from build123d import *

# Parameters (mm, degrees)
SKETCH_R  = 1.75
PAD_DEPTH = 9
FILLET_R  = 2


with BuildPart() as part:
    # Sketch → Pad (new body)
    with BuildSketch(Plane.XY):
        with BuildLine():
            Line((-15, 16), (15, 16))
            ThreePointArc((19, 12), (17.828427, 14.828427), (15, 16))
            Line((19, 12), (19, -12))
            ThreePointArc((15, -16), (17.828427, -14.828427), (19, -12))
            Line((15, -16), (-15, -16))
            ThreePointArc((-19, -12), (-17.828427, -14.828427), (-15, -16))
            Line((-19, -12), (-19, 12))
            ThreePointArc((-15, 16), (-17.828427, 14.828427), (-19, 12))
        make_face()
        with Locations((-15, 12)):
            Circle(SKETCH_R, mode=Mode.SUBTRACT)
        with Locations((15, 12)):
            Circle(SKETCH_R, mode=Mode.SUBTRACT)
        with Locations((15, -12)):
            Circle(SKETCH_R, mode=Mode.SUBTRACT)
        with Locations((-15, -12)):
            Circle(SKETCH_R, mode=Mode.SUBTRACT)
        with BuildLine():
            Line((-16.75, 8), (-15, 8))
            ThreePointArc((-15, 8), (-12.171573, 9.171573), (-11, 12))
            Line((-11, 12), (-11, 13.75))
            Line((-11, 13.75), (11, 13.75))
            Line((11, 13.75), (11, 12))
            ThreePointArc((11, 12), (12.171573, 9.171573), (15, 8))
            Line((15, 8), (16.75, 8))
            Line((16.75, 8), (16.75, -8))
            Line((15, -8), (16.75, -8))
            ThreePointArc((15, -8), (12.171573, -9.171573), (11, -12))
            Line((11, -13.75), (11, -12))
            Line((11, -13.75), (-11, -13.75))
            Line((-11, -12), (-11, -13.75))
            ThreePointArc((-11, -12), (-12.171573, -9.171573), (-15, -8))
            Line((-16.75, -8), (-15, -8))
            Line((-16.75, -8), (-16.75, 8))
        make_face(mode=Mode.SUBTRACT)
    extrude(amount=PAD_DEPTH)

    # Fillet
    fillet_edges = [part.edges().sort_by_distance(p)[0] for p in [
        (-11, 13.75, 4.5),
        (-16.75, 8, 4.5),
        (11, 13.75, 4.5),
        (16.75, 8, 4.5),
        (16.75, -8, 4.5),
        (11, -13.75, 4.5),
        (-11, -13.75, 4.5),
        (-16.75, -8, 4.5),
    ]]
    fillet(fillet_edges, radius=FILLET_R)


solid = part.part
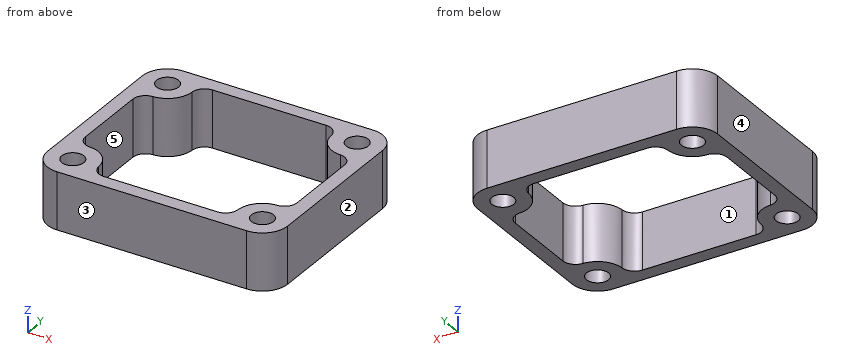
Work out the finished part from the listing and answer in its coordinate system (mm). Face numbers are marked on the shaded views. A direction names the side the tool comes from. Round coordinates to 2 decimals unless told otherwise and drop trailing zeros. Write each loop counter-clockwise with the first axis right and the second up, starting at its lowest first coordinate (ties: lowest second). Pieces come first, ordered by that corner, then holes. Notation, with made-up numbers: M -40,60.5 L -15,60.5 A34 cw -15,91.5 Z; hole C 88,15 d8. An arc over 180 degrees is marked long. Use a Markdown table: item, result.
1) Which of the six approach directions +Z, -Z, +X, -X, +Y, -Y give full straight-line access (tool end or side, diameter ignored) to the marked faces 1 and 2?
Taken from the geometry:
| item | result |
|---|---|
| face 1 | +Z, -Z |
| face 2 | +Z, -Z, +X, +Y, -Y |
2) The part is cut by section A-A on x = 7. Give the vertices of the cut face in (y, z), plus the area to 3 significant figures.
Taken from the geometry:
| item | result |
|---|---|
| outline | M -16,0 L -13.75,0 L -13.75,9 L -16,9 Z; M 13.75,0 L 16,0 L 16,9 L 13.75,9 Z |
| area | 40.5 mm2 |
3) The part is cut by section B-B on y = 3. Give the vertices of the cut face in (x, z).
Taken from the geometry:
| item | result |
|---|---|
| outline | M -19,0 L -16.75,0 L -16.75,9 L -19,9 Z; M 16.75,0 L 19,0 L 19,9 L 16.75,9 Z |
4) A flat-ended cylindrical pin translates along its axis: pin 1 (5 mm diameter, centred on x = 4, y = 11, fed in from -Z). Find the tip coordinate at first contact, or state that the pin passes through.
Taken from the geometry:
| item | result |
|---|---|
| pin 1 | passes through |
5) The part is cut by section D-D on z = 4.5. State how many separate pieces and enclosed holes the cut face has, plus the area to 3 significant figures.
Taken from the geometry:
| item | result |
|---|---|
| separate pieces | 1 |
| enclosed holes | 5 |
| area | 368 mm2 |
6) Determine the mould class of the marked faces 3, 4 and 5 for opening direction X: pulls with the +X half, pulls with the -X half, needs draft (parallel to the pull), parting line crosses it, or undercut.
Taken from the geometry:
| item | result |
|---|---|
| face 3 | needs draft |
| face 4 | pulls with the -X half |
| face 5 | undercut |
7) Consider line 1 (X direction, y = 5, z = 5.5); line 2 (Y direction, x = -3.5, z = 0.5); line 3 (Y direction, x = -15, z = 7.25). Determine where each line is inside the solid, lowest interval first. Write a range as [from, to].
Taken from the geometry:
| item | result |
|---|---|
| line 1 | x = [-19, -16.75], [16.75, 19] |
| line 2 | y = [-16, -13.75], [13.75, 16] |
| line 3 | y = [-16, -13.75], [-10.25, -7.99], [7.99, 10.25], [13.75, 16] |
8) The part is cut by section C-C on y = -11. Give the vertices of the cut face in (x, z).
Taken from the geometry:
| item | result |
|---|---|
| outline | M -19,0 L -16.44,0 L -16.44,9 L -19,9 Z; M -13.56,0 L -11.13,0 L -11.13,9 L -13.56,9 Z; M 11.13,0 L 13.56,0 L 13.56,9 L 11.13,9 Z; M 16.44,0 L 19,0 L 19,9 L 16.44,9 Z |
